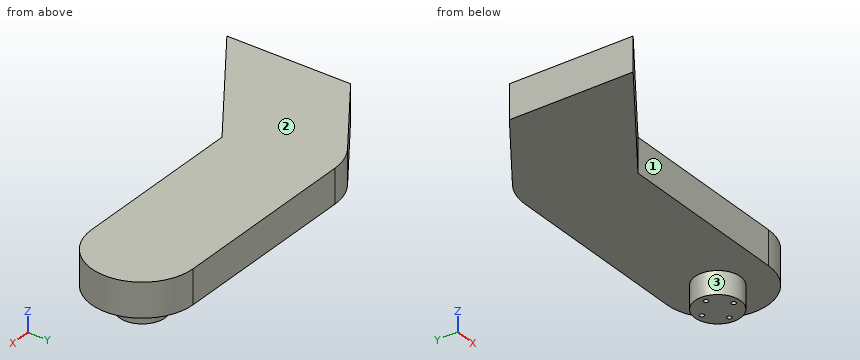
from build123d import *

# Parameters (mm, degrees)
SKETCH_1_W          = 300
SKETCH_1_H          = 44.73
EXTRUDE_1_DEPTH     = 15
CUT_EXTRUDE_4_REACH = 305.687
SKETCH_6_R          = 10
EXTRUDE_2_DEPTH     = 10
SKETCH_7_R          = 1
CUT_EXTRUDE_6_DEPTH = 5
EXTRUDE_START       = 15
EXTRUDE_5_DEPTH     = 15
CUT_EXTRUDE_7_DEPTH = 15


with BuildPart() as part:
    # 草图1 → 凸台-拉伸1 (new body)
    with BuildSketch(Plane.XY):
        with Locations((150, 22.365)):
            Rectangle(SKETCH_1_W, SKETCH_1_H)
    extrude(amount=EXTRUDE_1_DEPTH)

    # 草图4 → 切除-拉伸4 (cut, up to next)
    with BuildSketch(Plane.XY.offset(15), mode=Mode.PRIVATE) as cut_extrude_4_sk1:
        with BuildLine():
            Line((300, 44.73), (153.211623388, 44.73))
            ThreePointArc((153.211623388, 44.73), (175.576623388, 22.365), (153.211623388, 0))
            Line((153.211623388, 0), (300, 0))
            Line((300, 0), (300, 44.73))
        make_face()
    cut_extrude_4_tool1 = extrude(cut_extrude_4_sk1.sketch, amount=-CUT_EXTRUDE_4_REACH, mode=Mode.PRIVATE) & part.part
    add(cut_extrude_4_tool1.solids().sort_by_distance((235.292113, 22.365, 15))[0], mode=Mode.SUBTRACT)

    # 草图6 → 凸台-拉伸2 (add)
    with BuildSketch(Plane(origin=(0, 0, 0), x_dir=(-1, 0, 0), z_dir=(0, 0, -1))):
        with Locations((-153.211623388, 22.365)):
            Circle(SKETCH_6_R)
    extrude(amount=EXTRUDE_2_DEPTH)

    # 草图7 → 切除-拉伸6 (cut)
    with BuildSketch(Plane(origin=(0, 0, -10), x_dir=(-1, 0, 0), z_dir=(0, 0, -1))):
        with Locations((-153.211623388, 29.365)):
            Circle(SKETCH_7_R)
        with Locations((-146.211623388, 22.365)):
            Circle(SKETCH_7_R)
        with Locations((-153.211623388, 15.365)):
            Circle(SKETCH_7_R)
        with Locations((-160.211623388, 22.365)):
            Circle(SKETCH_7_R)
    extrude(amount=-CUT_EXTRUDE_6_DEPTH, mode=Mode.SUBTRACT)

    # 草图9 → 凸台-拉伸5 (add)
    # profile 1 of 8: a face of its own
    with BuildSketch(Plane.XY.offset(EXTRUDE_START)):
        with BuildLine():
            ThreePointArc((49.891287917, 9.536963001), (46.186397992, 26.248641494), (55.383586389, 40.685335471))
            Line((55.383586389, 40.685335471), (19.062500731, 15.253037497))
            Line((19.062500731, 15.253037497), (19.062500731, -12.049586181))
            Line((19.062500731, -12.049586181), (49.891287917, 9.536963001))
        make_face()
    # profile 2 of 8: a face of its own
    with BuildSketch(Plane.XY.offset(EXTRUDE_START)):
        with BuildLine():
            ThreePointArc((68.211623388, 0), (57.884615653, 2.527002716), (49.891287917, 9.536963001))
            Line((49.891287917, 9.536963001), (19.062500731, -12.049586181))
            Line((19.062500731, -12.049586181), (19.062500731, -39.352209859))
            Line((19.062500731, -39.352209859), (75.263280801, 0))
            Line((75.263280801, 0), (68.211623388, 0))
        make_face()
    # profile 3 of 8: a face of its own
    with BuildSketch(Plane.XY.offset(EXTRUDE_START)):
        with BuildLine():
            ThreePointArc((90.576623388, 22.365), (84.026066549, 38.179443161), (68.211623388, 44.73))
            ThreePointArc((68.211623388, 44.73), (61.486338182, 43.694879603), (55.383586389, 40.685335471))
            ThreePointArc((55.383586389, 40.685335471), (46.186397992, 26.248641494), (49.891287917, 9.536963001))
            Line((49.891287917, 9.536963001), (68.211623388, 22.365))
            Line((68.211623388, 22.365), (90.576623388, 22.365))
        make_face()
    # profile 4 of 8: a face of its own
    with BuildSketch(Plane.XY.offset(EXTRUDE_START)):
        with BuildLine():
            ThreePointArc((81.039660387, 4.044664529), (88.049620672, 12.037992265), (90.576623388, 22.365))
            Line((90.576623388, 22.365), (68.211623388, 22.365))
            Line((68.211623388, 22.365), (49.891287917, 9.536963001))
            ThreePointArc((49.891287917, 9.536963001), (57.884615653, 2.527002716), (68.211623388, 0))
            ThreePointArc((68.211623388, 0), (74.936908594, 1.035120397), (81.039660387, 4.044664529))
        make_face()
    # profile 5 of 8: a face of its own
    with BuildSketch(Plane.XY.offset(EXTRUDE_START)):
        with BuildLine():
            ThreePointArc((153.211623388, 0), (137.397180227, 6.550556839), (130.846623388, 22.365))
            Line((130.846623388, 22.365), (90.576623388, 22.365))
            ThreePointArc((90.576623388, 22.365), (88.049620672, 12.037992265), (81.039660387, 4.044664529))
            Line((81.039660387, 4.044664529), (75.263280801, 0))
            Line((75.263280801, 0), (153.211623388, 0))
        make_face()
    # profile 6 of 8: a face of its own
    with BuildSketch(Plane.XY.offset(EXTRUDE_START)):
        with BuildLine():
            ThreePointArc((130.846623388, 22.365), (137.397180227, 38.179443161), (153.211623388, 44.73))
            Line((153.211623388, 44.73), (68.211623388, 44.73))
            ThreePointArc((68.211623388, 44.73), (84.026066549, 38.179443161), (90.576623388, 22.365))
            Line((90.576623388, 22.365), (130.846623388, 22.365))
        make_face()
    # profile 7 of 8: a face of its own
    with BuildSketch(Plane.XY.offset(EXTRUDE_START)):
        with BuildLine():
            ThreePointArc((175.576623388, 22.365), (169.026066549, 38.179443161), (153.211623388, 44.73))
            ThreePointArc((153.211623388, 44.73), (137.397180227, 38.179443161), (130.846623388, 22.365))
            ThreePointArc((130.846623388, 22.365), (137.397180227, 6.550556839), (153.211623388, 0))
            ThreePointArc((153.211623388, 0), (169.026066549, 6.550556839), (175.576623388, 22.365))
        make_face()
        with BuildLine():
            ThreePointArc((163.211623388, 22.365), (153.211623388, 12.365), (143.211623388, 22.365))
            ThreePointArc((143.211623388, 22.365), (153.211623388, 32.365), (163.211623388, 22.365))
        make_face(mode=Mode.SUBTRACT)
    # profile 8 of 8: a face of its own
    with BuildSketch(Plane.XY.offset(EXTRUDE_START)):
        with BuildLine():
            Line((75.263280801, 0), (81.039660387, 4.044664529))
            ThreePointArc((81.039660387, 4.044664529), (74.936908594, 1.035120397), (68.211623388, 0))
            Line((68.211623388, 0), (75.263280801, 0))
        make_face()
    extrude(amount=-EXTRUDE_5_DEPTH)

    # 草图10 → 切除-拉伸7 (cut)
    with BuildSketch(Plane(origin=(0, 0, 0), x_dir=(-1, 0, 0), z_dir=(0, 0, -1))):
        with BuildLine():
            Line((-19.062500731, 15.253037497), (-19.062500731, 0))
            Line((-19.062500731, 0), (0, 0))
            Line((0, 0), (0, 44.73))
            Line((0, 44.73), (-68.211623388, 44.73))
            ThreePointArc((-68.211623388, 44.73), (-61.486338182, 43.694879603), (-55.383586389, 40.685335471))
            Line((-55.383586389, 40.685335471), (-19.062500731, 15.253037497))
        make_face()
    extrude(amount=-CUT_EXTRUDE_7_DEPTH, mode=Mode.SUBTRACT)


solid = part.part
Source: CAD feature listing. Evaluate the final solid. Frame: model axes, mm. Face numbers are marked on the shaded views. A direction names the side the tool comes from. Round coordinates to 2 decimals unless told otherwise and drop trailing zeros. Loops run counter-clockwise (first coordinate to the right, second up) from the corner with the lowest first, then second, coordinate; pieces in that order, holes last. Notation, with made-up numbers: M -5,24.25 L 26,24.25 A4 ccw 26,30.25 Z; hole C 56.5,-37.5 d5. An arc over 180 degrees is marked long. Return JSON: item names as keys, results as strings. Group by question number.
1. Section query D-D on z = -3.25. Output: boundary loops of the cut face in (x, y) (3 decimals).
2. Section query B-B on x = 110. Output: boundary loops of the cut face in (y, z).
3. Section query C-C on y = -5.5. Output: boundary loops of the cut face in (x, z).
4. Reachability of the marked faces 1, 2 and 3 from +Z, -Z, +X, -X, +Y, -Y: full face, straight path, thin tool, end or side. Return the list, or none.
5. Material intervals for line 1 along Z through (x, y) = (107.5, 35); line 2 along Y through (x, z) = (38, 13); line 3 along X through (y, z) = (25.5, -2.5), sorted ascending. Write a range as from..to.
6. Pin query (flat end, axial travel): pin 1 (1 mm diameter, centred on x = 153.5, y = 29.5, fed in from -Z); pin 2 (2 mm diameter, centred on x = 160.5, y = 22.5, fed in from -Z); pin 3 (8 mm diameter, centred on x = 72, z = -7, fed in from -Y); pin 4 (10 mm diameter, centred on x = 113, z = 4, fed in from -Y). Return the tip coordinate at first contact, or that it passes through.
Checks:
{
 "1": {"outline": "C 153.212,22.365 d20"},
 "2": {"outline": "M 0,0 L 44.73,0 L 44.73,15 L 0,15 Z"},
 "3": {"outline": "M 19.06,0 L 67.41,0 L 67.41,15 L 19.06,15 Z"},
 "4": {"face 1": "+Z, -Z, +X, -Y", "face 2": "+Z, +X, -X, +Y, -Y", "face 3": "-Z"},
 "5": {"line 1": "z = 0..15", "line 2": "y = -26.09..28.51", "line 3": "x = 143.72..162.71"},
 "6": {"pin 1": "stops at z = -5", "pin 2": "stops at z = -10", "pin 3": "passes through", "pin 4": "stops at y = 0"}
}
